```python
from build123d import *

# Parameters (mm, degrees)
SKETCH_1_W          = 290
SKETCH_1_H          = 925
EXTRUDE_1_DEPTH     = 12
EXTRUDE_3_DEPTH     = 12
EXTRUDE_4_DEPTH     = 300
CUT_EXTRUDE_1_DEPTH = 12
EXTRUDE_5_DEPTH     = 90
EXTRUDE_6_DEPTH     = 102
EXTRUDE_7_DEPTH     = 12


with BuildPart() as part:
    # 草图1 → 凸台-拉伸1 (new body)
    with BuildSketch(Plane(origin=(0, 0, 0), x_dir=(1, 0, 0), z_dir=(0, 1, 0))):
        with Locations((145, 462.5)):
            Rectangle(SKETCH_1_W, SKETCH_1_H)
    extrude(amount=EXTRUDE_1_DEPTH)

    # 草图3 → 凸台-拉伸3 (add)
    with BuildSketch(Plane(origin=(0, 12, 0), x_dir=(1, 0, 0), z_dir=(0, 1, 0))):
        Polygon((290, 330), (317.181818182, 330), (375, 270), (375, 53), (320, 0), (290, 0), align=None)
    extrude(amount=-EXTRUDE_3_DEPTH)

    # 草图4 → 凸台-拉伸4 (add)
    with BuildSketch(Plane(origin=(0, 12, 0), x_dir=(1, 0, 0), z_dir=(0, 1, 0))):
        Polygon((0, 925), (0, 0), (320, 0), (375, 53), (375, 270), (317.181818182, 330), (290, 330), (290, 925), align=None)
        Polygon((12, 913), (12, 12), (315.159103589, 12), (363, 58.101227451), (363, 265.159103589), (312.080590731, 318), (278, 318), (278, 913), align=None, mode=Mode.SUBTRACT)
    extrude(amount=EXTRUDE_4_DEPTH)

    # 草图5 → 切除-拉伸1 (cut)
    with BuildSketch(Plane(origin=(290, 0, 0), x_dir=(0, 0, -1), z_dir=(1, 0, 0))):
        Polygon((775, 312), (925, 47), (925, 312), align=None)
    extrude(amount=-CUT_EXTRUDE_1_DEPTH, mode=Mode.SUBTRACT)

    # 草图7 → 凸台-拉伸5 (add)
    with BuildSketch(Plane(origin=(290, 0, 0), x_dir=(0, 0, -1), z_dir=(1, 0, 0))):
        Polygon((775, 312), (925, 47), (925, 22.639376034), (761.210967567, 312), align=None)
    extrude(amount=EXTRUDE_5_DEPTH)

    # 草图8 → 凸台-拉伸6 (add)
    with BuildSketch(Plane(origin=(278, 0, 0), x_dir=(0, 0, -1), z_dir=(1, 0, 0))):
        Polygon((925, 312), (925, 47), (913, 68.2), (913, 312), align=None)
    extrude(amount=EXTRUDE_6_DEPTH)

    # 草图9 → 凸台-拉伸7 (add)
    with BuildSketch(Plane(origin=(380, 0, 0), x_dir=(0, 0, -1), z_dir=(1, 0, 0))):
        Polygon((761.210967567, 312), (925, 312), (925, 22.639376034), align=None)
    extrude(amount=EXTRUDE_7_DEPTH)


solid = part.part
```
Geometry: final body of the model. Coordinates: model frame, mm. A direction names the side the tool comes from. Coordinates: 2 decimals unless noted, no trailing zeros. Order: outer loops, then holes, each group sorted by start corner. A loop starts at its lowest first (then second) coordinate and runs counter-clockwise, first axis right, second up.
Item 1: Draft query along X for faces 1 (the face through (347.115, 153.816, -26.129)), 2 (the face through (193, 158, -925)), 3 (the face through (328.29, 191.81, -843.03)). Return one class per face: released by +X, released by -X, zero draft, split by the parting line, or undercut.
Answer:
face 1: released by +X
face 2: zero draft
face 3: undercut
Item 2: Section query A-A (z = -86). Output: boundary loops of the cut face in (x, y).
Answer:
outline: (0, 0) - (375, 0) - (375, 312) - (363, 312) - (363, 12) - (12, 12) - (12, 312) - (0, 312) - close
Item 3: Contact query for flat-ended pins moving along their axis: P1, Ø12, axis at x = 112.5, z = -384.5, coming from the +Y side; P2, Ø4, axis at y = 88.5, z = -714, coming from the +X side. Output: stop coordinate, or through.
Answer:
P1: stops at y = 12
P2: stops at x = 290
Item 4: Access query for faces 4 (the face through (193, 160, -913)), 5 (the face through (340.286, 165.294, -844.252)), 6 (the face through (375, 154, -160)). Directions: +Z, -Z, +X, -X, +Y, -Y. A direction counts if a zero-diameter tool reaches every point of the face in a straight line with its end or side. Return the directions, or none.
Answer:
face 4: +Y
face 5: +X, -Y
face 6: +Z, +X, +Y, -Y
Item 5: Section query C-C (y = 242). Output: boundary loops of the cut face in (x, z).
Answer:
outline: (0, -925) - (392, -925) - (392, -800.83) - (290, -800.83) - (290, -330) - (317.18, -330) - (375, -270) - (375, -53) - (320, 0) - (0, 0) - close; hole (12, -913) - (380, -913) - (380, -814.62) - (278, -814.62) - (278, -318) - (312.08, -318) - (363, -265.16) - (363, -58.1) - (315.16, -12) - (12, -12) - close
Item 6: Section query D-D (z = -821). Output: boundary loops of the cut face in (x, y).
Answer:
outline: (0, 0) - (290, 0) - (290, 206.37) - (392, 206.37) - (392, 312) - (380, 312) - (380, 230.73) - (278, 230.73) - (278, 12) - (12, 12) - (12, 312) - (0, 312) - close
Item 7: Section query B-B (x = 172). Output: boundary loops of the cut face in (y, z), then the cut area to 3 significant figures.
Answer:
outline: (0, -925) - (312, -925) - (312, -913) - (12, -913) - (12, -12) - (312, -12) - (312, 0) - (0, 0) - close
area: 18,300 mm2
Item 8: Material intervals for line 1 along Z through (x, y) = (232, 288); line 2 along X through (y, z) = (31.5, -404); line 3 along X through (y, z) = (166, -847), sorted ascending.
Answer:
line 1: z = -925 to -913, -12 to 0
line 2: x = 0 to 12, 278 to 290
line 3: x = 0 to 12, 278 to 392
